```python
from build123d import *

# Parameters (mm, degrees)
EXTRUDE_1_DEPTH     = 6.2
SKETCH_2_W          = 20
SKETCH_2_H          = 11.25
CUT_EXTRUDE_1_DEPTH = 4.4
CUT_EXTRUDE_2_DEPTH = 4.4
SKETCH_4_R          = 1
CUT_EXTRUDE_3_DEPTH = 21.169361046
SKETCH_5_R          = 2
CUT_EXTRUDE_4_DEPTH = 1.4
CUT_EXTRUDE_5_DEPTH = 4.4
CUT_EXTRUDE_6_DEPTH = 4.2


with BuildPart() as part:
    # Sketch 1 → Extrude 1 (new body)
    with BuildSketch(Plane(origin=(0, 0, 0), x_dir=(1, 0, 0), z_dir=(0, 1, 0))):
        with BuildLine():
            Line((-15.85, -5.625), (15.85, -5.625))
            Line((15.85, -5.625), (15.85, -2.13541565))
            ThreePointArc((15.85, -2.13541565), (17.05, 0), (15.85, 2.13541565))
            Line((15.85, 2.13541565), (15.85, 5.625))
            Line((15.85, 5.625), (-15.85, 5.625))
            Line((-15.85, 5.625), (-15.85, 2.5))
            ThreePointArc((-15.85, 2.5), (-18.35, 0), (-15.85, -2.5))
            Line((-15.85, -2.5), (-15.85, -5.625))
        make_face()
    extrude(amount=EXTRUDE_1_DEPTH)

    # Sketch 2 → Cut-Extrude 1 (cut)
    with BuildSketch(Plane.XZ):
        with Locations((-0.65, 0)):
            Rectangle(SKETCH_2_W, SKETCH_2_H)
    extrude(amount=-CUT_EXTRUDE_1_DEPTH, mode=Mode.SUBTRACT)

    # Sketch 3 → Cut-Extrude 2 (cut)
    with BuildSketch(Plane.XZ):
        with BuildLine():
            Line((-12.15, 4.625), (10.85, 4.625))
            ThreePointArc((10.85, 4.625), (11.557106781, 4.332106781), (11.85, 3.625))
            Line((11.85, 3.625), (11.85, -2.375))
            ThreePointArc((11.85, -2.375), (11.557106781, -3.082106781), (10.85, -3.375))
            Line((10.85, -3.375), (-12.15, -3.375))
            ThreePointArc((-12.15, -3.375), (-12.857106781, -3.082106781), (-13.15, -2.375))
            Line((-13.15, -2.375), (-13.15, 3.625))
            ThreePointArc((-13.15, 3.625), (-12.857106781, 4.332106781), (-12.15, 4.625))
        make_face()
    extrude(amount=-CUT_EXTRUDE_2_DEPTH, mode=Mode.SUBTRACT)

    # Sketch 4 → Cut-Extrude 3 (cut, through all)
    with BuildSketch(Plane(origin=(0, 6.2, 0), x_dir=(1, 0, 0), z_dir=(0, 1, 0))):
        with Locations(Location((-15.85, 0, 0), (0, 0, 270))):
            Circle(SKETCH_4_R)
        with Locations(Location((14.55, 0, 0), (0, 0, 270))):
            Circle(SKETCH_4_R)
    extrude(amount=-CUT_EXTRUDE_3_DEPTH, mode=Mode.SUBTRACT)

    # Sketch 5 → Cut-Extrude 4 (cut)
    with BuildSketch(Plane(origin=(0, 6.2, 0), x_dir=(1, 0, 0), z_dir=(0, 1, 0))):
        with Locations(Location((-15.85, 0, 0), (0, 0, 270))):
            Circle(SKETCH_5_R)
        with Locations(Location((14.55, 0, 0), (0, 0, 90))):
            Circle(SKETCH_5_R)
    extrude(amount=-CUT_EXTRUDE_4_DEPTH, mode=Mode.SUBTRACT)

    # Sketch 6 → Cut-Extrude 5 (cut)
    with BuildSketch(Plane.XZ):
        with BuildLine():
            Line((11.95, 3.625), (11.95, -2.375))
            ThreePointArc((11.95, -2.375), (11.627817459, -3.152817459), (10.85, -3.475))
            Line((10.85, -3.475), (-12.15, -3.475))
            ThreePointArc((-12.15, -3.475), (-12.927817459, -3.152817459), (-13.25, -2.375))
            Line((-13.25, -2.375), (-13.25, 3.625))
            ThreePointArc((-13.25, 3.625), (-12.927817459, 4.402817459), (-12.15, 4.725))
            Line((-12.15, 4.725), (10.85, 4.725))
            ThreePointArc((10.85, 4.725), (11.627817459, 4.402817459), (11.95, 3.625))
        make_face()
    extrude(amount=-CUT_EXTRUDE_5_DEPTH, mode=Mode.SUBTRACT)

    # Sketch 7 → Cut-Extrude 6 (cut)
    with BuildSketch(Plane.XZ.offset(-4.4)):
        with BuildLine():
            Line((-8.15, 3.125), (6.85, 3.125))
            ThreePointArc((6.85, 3.125), (9.35, 0.625), (6.85, -1.875))
            Line((6.85, -1.875), (-8.15, -1.875))
            ThreePointArc((-8.15, -1.875), (-10.65, 0.625), (-8.15, 3.125))
        make_face()
    extrude(amount=-CUT_EXTRUDE_6_DEPTH, mode=Mode.SUBTRACT)


solid = part.part
```
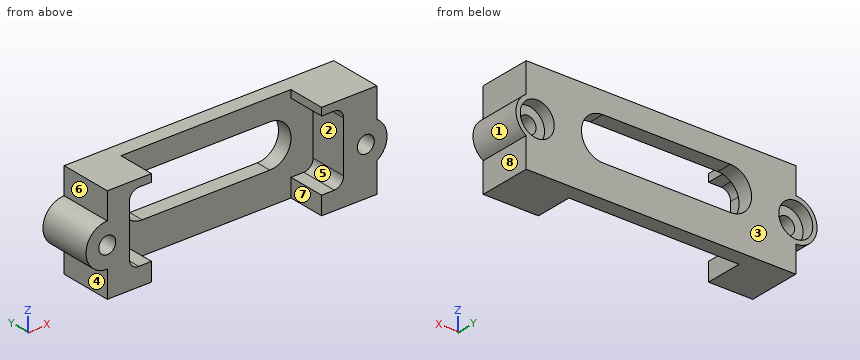
Can you work these out from the model? Positions are in its coordinate system, mm. Face numbers are marked on the shaded views. A direction names the side the tool comes from. Coordinates: 2 decimals unless noted, no trailing zeros. Order: outer loops, then holes, each group sorted by start corner. A loop starts at its lowest first (then second) coordinate and runs counter-clockwise, first axis right, second up. Notation, with made-up numbers: (23.5, 81) -> (55.5, 81) arc R21 ccw to (55.5, 119) -> close; hole circle Ø6 at (32.25, 3). An arc over 180 degrees is marked (long way). Write each question's results on one line, items separated by ' | '.
Item 1: If I drill on line 1 along X through (y, z) = (0.5, 0); line 2 along X through (y, z) = (1.75, 3.25); line 3 along X through (y, z) = (5.2, 0), over which ranges is the centre line in solid material (lowest first)?
Results are:
line 1: -18.35 to -16.85, -14.85 to -13.25, 11.95 to 13.55, 15.55 to 17.05 | line 2: -15.85 to -13.25, 11.95 to 15.85 | line 3: -18.35 to -17.85, -13.85 to -10.57, 9.27 to 12.55, 16.55 to 17.05
Item 2: I'm going to push flat-ended pins straight in: pin 1 Ø3 at (x, z) = (-15.85, 0) entering from +Y; pin 2 Ø1.7 at (y, z) = (3.5, -5) entering from -X; pin 3 Ø1.1 at (y, z) = (3, -5) entering from +X; pin 4 Ø6.5 at (x, z) = (-15.85, 0) entering from +Y. Where does each tip first touch, or does it pass through?
Results are:
pin 1: y = 4.8 | pin 2: x = -15.85 | pin 3: x = 15.85 | pin 4: y = 6.2
Item 3: I want a section at A-A, the plane y = 3.5. Write out the boundary of the cut face in (x, z) (3 decimals), then the cut area to 3 significant figures.
Results are:
outline: (-15.85, -5.625) -> (-10.65, -5.625) -> (-10.65, -3.475) -> (-12.15, -3.475) arc R1.1 cw to (-13.25, -2.375) -> (-13.25, 3.625) arc R1.1 cw to (-12.15, 4.725) -> (-10.65, 4.725) -> (-10.65, 5.625) -> (-15.85, 5.625) -> (-15.85, 2.5) arc R2.5 ccw to (-15.85, -2.5) -> close; (9.35, -5.625) -> (15.85, -5.625) -> (15.85, -2.135) arc R2.5 ccw to (15.85, 2.135) -> (15.85, 5.625) -> (9.35, 5.625) -> (9.35, 4.725) -> (10.85, 4.725) arc R1.1 cw to (11.95, 3.625) -> (11.95, -2.375) arc R1.1 cw to (10.85, -3.475) -> (9.35, -3.475) -> close; hole circle Ø2 at (-15.85, 0); hole circle Ø2 at (14.55, 0) | area: 97.2 mm²
Item 4: Which directions (+Z, -Z, +X, -X, +Y, -Y) give clear straight access to the entire face, cutting with the end or side of a thin tool? Please do the marked faces 5, 6, 7 and 8.
Results are:
face 5: -Y | face 6: +Z, -X, +Y, -Y | face 7: +Z, -Z, -Y | face 8: -Z, +X, +Y, -Y
Item 5: I want a section at C-C, the plane y = 5.75. Write out the boundary of the cut face in (x, z) (3 decimals), then the cut area to 3 significant figures.
Results are:
outline: (-15.85, -5.625) -> (15.85, -5.625) -> (15.85, -2.135) arc R2.5 ccw to (15.85, 2.135) -> (15.85, 5.625) -> (-15.85, 5.625) -> (-15.85, 2.5) arc R2.5 ccw to (-15.85, -2.5) -> close; hole circle Ø4 at (-15.85, 0); hole (-8.15, -1.875) -> (6.85, -1.875) arc R2.5 ccw to (6.85, 3.125) -> (-8.15, 3.125) arc R2.5 ccw to start; hole circle Ø4 at (14.55, 0) | area: 250 mm²
Item 6: I want a section at D-D, the plane z = 0.5. Write out the boundary of the cut face in (x, y), then the cut area to 3 significant figures.
Results are:
outline: (-18.3, 0) -> (-16.72, 0) -> (-16.72, 4.8) -> (-17.79, 4.8) -> (-17.79, 6.2) -> (-18.3, 6.2) -> close; (-14.98, 0) -> (-13.25, 0) -> (-13.25, 4.4) -> (-10.65, 4.4) -> (-10.65, 6.2) -> (-13.91, 6.2) -> (-13.91, 4.8) -> (-14.98, 4.8) -> close; (9.35, 4.4) -> (11.95, 4.4) -> (11.95, 0) -> (13.68, 0) -> (13.68, 4.8) -> (12.61, 4.8) -> (12.61, 6.2) -> (9.35, 6.2) -> close; (15.42, 0) -> (17, 0) -> (17, 6.2) -> (16.49, 6.2) -> (16.49, 4.8) -> (15.42, 4.8) -> close | area: 44.5 mm²
Item 7: If we mould it in two halves opening along X, with no side actions, what happens to the marked faces 1, 2, 3 and 4? For each: +X half, -X half, draft (parallel to the pull), parting line (faces both ways), or undercut.
Results are:
face 1: +X half | face 2: undercut | face 3: draft | face 4: -X half
Item 8: I want a section at B-B, the plane x = 3. Write out the boundary of the cut face in (y, z) (3 decimals), then the cut area to 4 significant figures.
Results are:
outline: (4.4, -5.625) -> (6.2, -5.625) -> (6.2, -1.875) -> (4.4, -1.875) -> close; (4.4, 3.125) -> (6.2, 3.125) -> (6.2, 5.625) -> (4.4, 5.625) -> close | area: 11.25 mm²
